from build123d import *

# Parameters (mm, degrees)
ESQUISSE1_W             = 54
ESQUISSE1_H             = 18
ESQUISSE1_R             = 3
BOSS_EXTRU_1_DEPTH      = 59
ESQUISSE2_W             = 89.885876072
ESQUISSE2_H             = 74.564815434
ENL_V_MAT_EXTRU_1_DEPTH = 13
ESQUISSE3_R             = 6
ENL_V_MAT_EXTRU_2_DEPTH = 13


with BuildPart() as part:
    # Esquisse1 → Boss.-Extru.1 (new body)
    with BuildSketch(Plane.XY):
        Rectangle(ESQUISSE1_W, ESQUISSE1_H)
        with Locations((-19, 2)):
            Circle(ESQUISSE1_R, mode=Mode.SUBTRACT)
        with Locations((21, 2)):
            Circle(ESQUISSE1_R, mode=Mode.SUBTRACT)
    extrude(amount=BOSS_EXTRU_1_DEPTH)

    # Esquisse2 → Enlèv. mat.-Extru.1 (cut)
    with BuildSketch(Plane(origin=(0, 9, 0), x_dir=(1, 0, 0), z_dir=(0, 1, 0))):
        with Locations((-2.437014962, -42.282407717)):
            Rectangle(ESQUISSE2_W, ESQUISSE2_H)
    extrude(amount=-ENL_V_MAT_EXTRU_1_DEPTH, mode=Mode.SUBTRACT)

    # Esquisse3 → Enlèv. mat.-Extru.2 (cut)
    with BuildSketch(Plane(origin=(0, -4, 0), x_dir=(1, 0, 0), z_dir=(0, 1, 0))):
        with Locations(Location((0, -46.74, 0), (0, 0, 270))):
            Circle(ESQUISSE3_R)
    extrude(amount=-ENL_V_MAT_EXTRU_2_DEPTH, mode=Mode.SUBTRACT)


solid = part.part
Input: part model. Units: mm. Frame: model coordinates. A direction names the side the tool comes from. Round coordinates to 2 decimals unless told otherwise and drop trailing zeros. Write each loop counter-clockwise with the first axis right and the second up, starting at its lowest first coordinate (ties: lowest second). Pieces come first, ordered by that corner, then holes.
1) Contact query for flat-ended pins moving along their axis: P1, Ø1.5, axis at x = -17, z = 36, coming from the +Y side; P2, Ø1.5, axis at x = 8, y = 0, coming from the +Z side. Output: stop coordinate, or through.
2) Reachability of faces 4 (the cylindrical face through (-22, 2, 2)), 5 (the flat face through (0, -4, 32)) from +Z, -Z, +X, -X, +Y, -Y: full face, straight path, thin tool, end or side. Return the list, or none.
3) Cut plane B-B (x = 0). Return the cut outline in (y, z).
4) Cut plane C-C (y = 2). Return the cut outline in (x, z).
5) Cut plane D-D (x = -10). Return the cut outline in (y, z).
6) Draft query along Y for faces 1 (the flat face through (0, 3, 5)), 2 (the cylindrical face through (18, 2, 2)), 3 (the flat face through (0, 9, 2)). Return one class per face: pulls with the +Y half, pulls with the -Y half, needs draft (parallel to the pull), parting line crosses it, or undercut.
7) Ray query, L1, parallel to X at y = 2, z = 1.8; L2, parallel to Y at x = 21, z = 1; L3, parallel to X at y = -6.7, z = 46.74. Return the intervals inside material, ascending.
8) Cut plane A-A (z = 46.74). Return the cut outline in (x, y).
Geometry says:
1. P1: stops at y = -4
1. P2: stops at z = 5
2. face 4: +Z, -Z
2. face 5: +Z, +X, -X, +Y
3. outline: (-9, 0) - (9, 0) - (9, 5) - (-4, 5) - (-4, 40.74) - (-9, 40.74) - close; (-9, 52.74) - (-4, 52.74) - (-4, 59) - (-9, 59) - close
4. outline: (-27, 0) - (-22, 0) - (-22, 5) - (-27, 5) - close; (-16, 0) - (18, 0) - (18, 5) - (-16, 5) - close; (24, 0) - (27, 0) - (27, 5) - (24, 5) - close
5. outline: (-9, 0) - (9, 0) - (9, 5) - (-4, 5) - (-4, 59) - (-9, 59) - close
6. face 1: needs draft
6. face 2: undercut
6. face 3: pulls with the +Y half
7. L1: x = -27 to -22, -16 to 18, 24 to 27
7. L2: y = -9 to -1, 5 to 9
7. L3: x = -27 to -6, 6 to 27
8. outline: (-27, -9) - (-6, -9) - (-6, -4) - (-27, -4) - close; (6, -9) - (27, -9) - (27, -4) - (6, -4) - close
